The figure shows three views and two pictorial views of one solid part (mm, origin at its lowest corner). Answer the questions. A direction names the side the tool comes from. Coordinates: 2 decimals unless noted, no trailing zeros. Write each loop counter-clockwise with the first axis right and the second up, starting at its lowest first coordinate (ties: lowest second). Pieces come first, ordered by that corner, then holes.
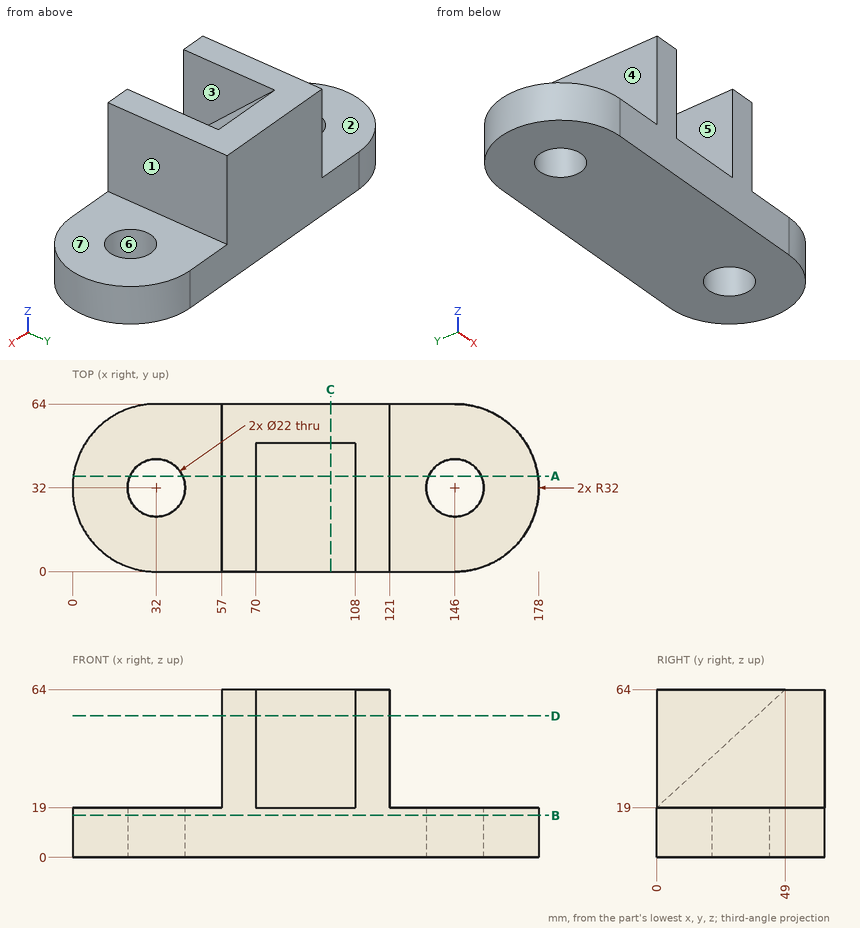
1. Section B-B on z = 16 is taken. Give the vertices of the cut face in (x, y).
Results found:
outline: (32, 0) - (146, 0) arc R32 ccw to (146, 64) - (32, 64) arc R32 ccw to start; hole circle Ø22 at (32, 32); hole circle Ø22 at (146, 32)
2. A tool of negligible diameter and unlimited length cuts with its end or side. For the marked faces 1, 2 and 3, from which of +Z, -Z, +X, -X, +Y, -Y can it reach the whole face along a straight path? Write none if from no direction.
Results found:
face 1: +Z, +X, +Y, -Y
face 2: +Z, -X, +Y, -Y
face 3: +Z, -Y
3. For a pull along X with two mould halves and no side action, classify the marked faces 4, 5, 6 and 7 as pulls with the +X half, pulls with the -X half, needs draft (parallel to the pull), parting line crosses it, or undercut.
Results found:
face 4: pulls with the -X half
face 5: undercut
face 6: undercut
face 7: needs draft
4. Section A-A on y = 36.5 is taken. Give the vertices of the cut face in (x, z), then the cut area to 3 significant figures.
Results found:
outline: (0.32, 0) - (21.96, 0) - (21.96, 19) - (0.32, 19) - close; (42.04, 0) - (135.96, 0) - (135.96, 19) - (121, 19) - (121, 64) - (108, 64) - (108, 52.52) - (70, 52.52) - (70, 64) - (57, 64) - (57, 19) - (42.04, 19) - close; (156.04, 0) - (177.68, 0) - (177.68, 19) - (156.04, 19) - close
area: 5,050 mm2
5. Section C-C on x = 98.5 is taken. Give the vertices of the cut face in (y, z).
Results found:
outline: (0, 0) - (64, 0) - (64, 64) - (49, 64) - (0, 19) - close
6. Section D-D on z = 54 is taken. Give the vertices of the cut face in (x, y), then the cut area to 3 significant figures.
Results found:
outline: (57, 0) - (70, 0) - (70, 38.11) - (108, 38.11) - (108, 0) - (121, 0) - (121, 64) - (57, 64) - close
area: 2,650 mm2
7. Flat-ended cylindrical pins translate along their axes: P1, Ø5, axis at y = 14.5, z = 44.5, coming from the +X side; P2, Ø1.5, axis at x = 61.5, y = 38, coming from the -Z side; P3, Ø1.5, axis at y = 31.5, z = 11, coming from the -X side; P4, Ø2, axis at y = 12, z = 57, coming from the -X side. Find the tip coordinate at first contact, or state that the pin passes through.
Results found:
P1: stops at x = 121
P2: stops at z = 0
P3: stops at x = 0
P4: stops at x = 57
8. Find the intervals of material crossed by L1, parallel to X at y = 32.5, z = 3.5; L2, parallel to Y at x = 146, z = 9.5; L3, parallel to X at y = 31, z = 49, in increasing order.
Results found:
L1: x = 0 to 21.01, 42.99 to 135.01, 156.99 to 178
L2: y = 0 to 21, 43 to 64
L3: x = 57 to 70, 108 to 121
